Check sheet for the drawn part. Datum: minimum x, y, z corner. Units: mm. A direction names the side the tool comes from. Give positions to 0.01 mm unless a question says otherwise; leave off trailing zeros. Order: outer loops, then holes, each group sorted by start corner. A loop starts at its lowest first (then second) coordinate and runs counter-clockwise, first axis right, second up. Notation, with made-up numbers: (-25.5, -8) -> (25.5, -8) arc R17 cw to (25.5, 15) -> close; hole circle Ø7 at (-20.5, 17). An arc over 180 degrees is marked (long way). Return JSON: item names as keys, results as strings. Group by question number.
(1) Release check for a two-part mould opening along Y. For the marked faces 1, 2 and 3 record: pulls with the +Y half, pulls with the -Y half, needs draft (parallel to the pull), parting line crosses it, or undercut.
(2) Depth check by flat-ended pin: pin 1 Ø1.5 at (x, y) = (5.5, 3) entering from +Z; pin 2 Ø1.5 at (x, z) = (4.5, 1.5) entering from +Y; pin 3 Ø1 at (x, y) = (8, 3.5) entering from +Z. Enter the tip coordinate at first touch or a pass-through.
(3) Tool access check on the marked faces 4, 5 and 6. Record the directions out of +Z, -Z, +X, -X, +Y, -Y that give a thin tool (end or side, any length) a straight path to the whole face; none if there is none.
(4) Cross-section at A-A on x = 4.75. Enter the section's corners in (y, z).
(5) Thickness scan on line 1 along X through (y, z) = (2.1, 0.55); line 2 along Y through (x, z) = (5.25, 2.25); line 3 along Y through (x, z) = (11.75, 1.5). Record the ranges inside material, lowest first.
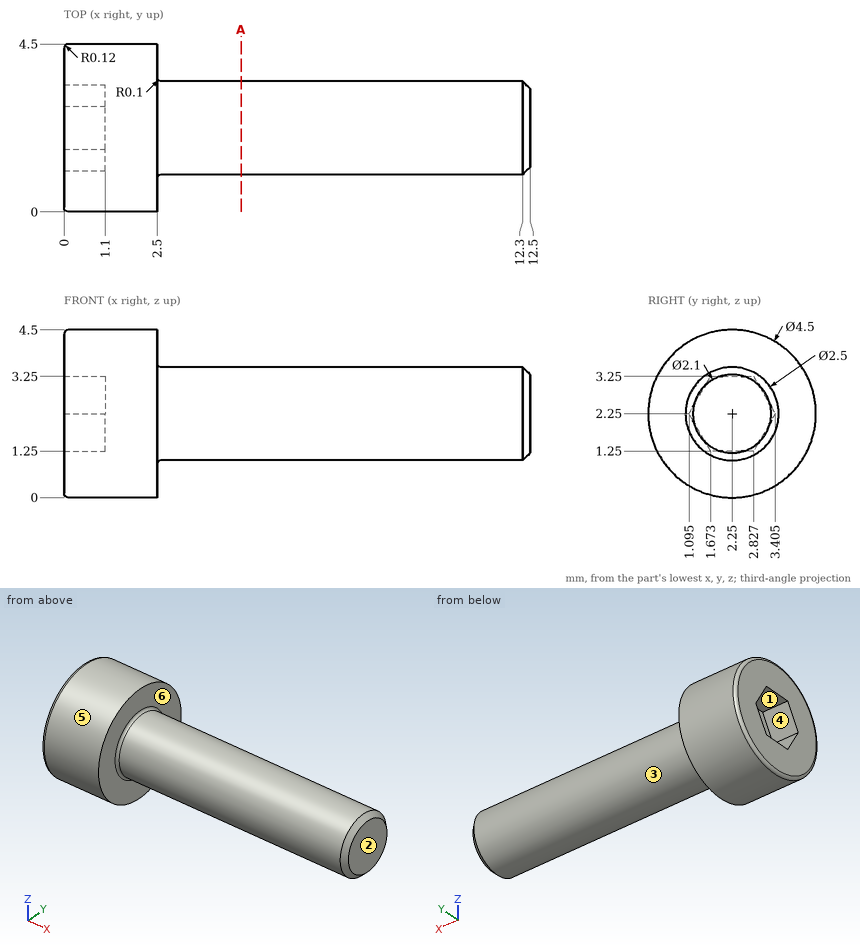
Verdict:
{
 "1": {"face 1": "undercut", "face 2": "needs draft", "face 3": "parting line crosses it"},
 "2": {"pin 1": "z = 3.5", "pin 2": "y = 3.5", "pin 3": "z = 3.25"},
 "3": {"face 4": "-X", "face 5": "+X, -X", "face 6": "+X"},
 "4": {"outline": "circle Ø2.5 at (2.25, 2.25)"},
 "5": {"line 1": "0 to 2.5", "line 2": "1 to 3.5", "line 3": "1.25 to 3.25"}
}
